Here's how the part is built. I have some questions about the finished solid (model axes, mm). Give positions to 0.01 mm unless a question says otherwise; leave off trailing zeros. Loops run counter-clockwise (first coordinate to the right, second up) from the corner with the lowest first, then second, coordinate; pieces in that order, holes last.
Q1. If we section it at D-D (x = -3.25): Please give me the cut outline in (y, z), plus the area to 3 significant figures.
Q2. We'd pull the mould along X, two halves only. Please class faces 1 (the face through (-10, 0, 0)), 2 (the face through (-0.56, -12.46, 0.04)), 3 (the face through (8, 19, 0)): +X half, -X half, draft (parallel to the pull), parting line (faces both ways), or undercut.
Q3. If we section it at A-A (y = 0): Please give me the cut outline in (x, z).
Q4. If we section it at B-B (x = 0): Please give me the cut outline in (y, z).
Q5. Will this pin go through, and if not, where does the flat tip stop? P1, Ø6, axis at x = 0, y = -15, coming from the -Z side.
Q6. If we section it at C-C (z = -1.9): Please give me the cut outline in (x, y), plus the area to 3 significant figures.
Q7. I need wall thicknesses on line 1 (Y direction, x = 0, z = 1.35); line 2 (Y direction, x = 3.25, z = 2.1); line 3 (X direction, y = -15, z = -1.3). Which ranges of each line are inside material? Lowest first, please.
from build123d import *

# Parameters (mm, degrees)
ESBO_O1_W                = 20
ESBO_O1_H                = 40
RESSALTO_EXTRUS_O1_DEPTH = 2.5
ESBO_O2_R                = 4.1
CORTE_EXTRUS_O1_DEPTH    = 23.912878475
ESBO_O3_R                = 2.6
CORTE_EXTRUS_O2_DEPTH    = 23.912878475
FILETE1_R                = 5


with BuildPart() as part:
    # Esboço1 → Ressalto-extrusão1 (new, symmetric)
    with BuildSketch(Plane.XY):
        Rectangle(ESBO_O1_W, ESBO_O1_H)
    extrude(amount=RESSALTO_EXTRUS_O1_DEPTH, both=True)

    # Esboço2 → Corte-extrusão1 (cut, through all)
    with BuildSketch(Plane.XY.offset(2.5)):
        Circle(ESBO_O2_R)
    extrude(amount=-CORTE_EXTRUS_O1_DEPTH, mode=Mode.SUBTRACT)

    # Esboço3 → Corte-extrusão2 (cut, through all)
    with BuildSketch(Plane.XY.offset(2.5)):
        with Locations((0, 15)):
            Circle(ESBO_O3_R)
    corte_extrus_o2 = extrude(amount=-CORTE_EXTRUS_O2_DEPTH, mode=Mode.SUBTRACT)

    # Espelhar1: Corte-extrusão2 across plane
    add(corte_extrus_o2.mirror(Plane.ZX), mode=Mode.SUBTRACT)

    # Filete1
    filete1_edges = [part.edges().sort_by_distance(p)[0] for p in [
        (10, -20, 0),
        (-10, -20, 0),
        (-10, 20, 0),
        (10, 20, 0),
    ]]
    fillet(filete1_edges, radius=FILETE1_R)


solid = part.part
Check sheet entries:
1. outline: (-20, -2.5) - (-2.5, -2.5) - (-2.5, 2.5) - (-20, 2.5) - close; (2.5, -2.5) - (20, -2.5) - (20, 2.5) - (2.5, 2.5) - close
1. area: 175 mm2
2. face 1: -X half
2. face 2: undercut
2. face 3: +X half
3. outline: (-10, -2.5) - (-4.1, -2.5) - (-4.1, 2.5) - (-10, 2.5) - close; (4.1, -2.5) - (10, -2.5) - (10, 2.5) - (4.1, 2.5) - close
4. outline: (-20, -2.5) - (-17.6, -2.5) - (-17.6, 2.5) - (-20, 2.5) - close; (-12.4, -2.5) - (-4.1, -2.5) - (-4.1, 2.5) - (-12.4, 2.5) - close; (4.1, -2.5) - (12.4, -2.5) - (12.4, 2.5) - (4.1, 2.5) - close; (17.6, -2.5) - (20, -2.5) - (20, 2.5) - (17.6, 2.5) - close
5. P1: stops at z = -2.5
6. outline: (-10, -15) arc R5 ccw to (-5, -20) - (5, -20) arc R5 ccw to (10, -15) - (10, 15) arc R5 ccw to (5, 20) - (-5, 20) arc R5 ccw to (-10, 15) - close; hole circle Ø8.2 at (0, 0); hole circle Ø5.2 at (0, -15); hole circle Ø5.2 at (0, 15)
6. area: 683 mm2
7. line 1: y = -20 to -17.6, -12.4 to -4.1, 4.1 to 12.4, 17.6 to 20
7. line 2: y = -20 to -2.5, 2.5 to 20
7. line 3: x = -10 to -2.6, 2.6 to 10
